Source: CAD feature listing. Evaluate the final solid. Frame: model axes, mm. A direction names the side the tool comes from. Round coordinates to 2 decimals unless told otherwise and drop trailing zeros. Loops run counter-clockwise (first coordinate to the right, second up) from the corner with the lowest first, then second, coordinate; pieces in that order, holes last.
(1) Section D-D, the plane x = 2.5. Return the cut outline in (y, z), plus the area to 3 significant figures.
(2) Section A-A, the plane y = 2. Return the cut outline in (x, z).
(3) Section C-C, the plane y = 3.25. Count the separate pieces of the cut face and the enclosed holes in it, plus the area to 3 significant figures.
(4) Section B-B, the plane z = -0.25. Return the cut outline in (x, y).
(5) Mould query, pull axis Z, two halves, no side actions, for faces 5 (the flat face through (6, 4, 0)), 6 (the flat face through (12, 4, 3)), 7 (the flat face through (1, 0, 3)). Classes: pulls with the +Z half, pulls with the -Z half, needs draft (parallel to the pull), parting line crosses it, or undercut.
(6) First-contact query: pin 1 Ø0.5 at (x, y) = (2.5, 4) entering from +Z; pin 2 Ø3 at (x, y) = (7.5, 6) entering from -Z; pin 3 Ø0.8 at (x, z) = (1, 3.5) entering from -Y. Flat tips, straight axial feed; report the tip coordinate or a pass-through.
(7) Material intervals for probe 1 along Z at (x, y) = (10, 1.25); probe 2 along X at (y, z) = (2, 3.5); probe 3 along Z at (x, y) = (11.5, 6), sorted ascending.
(8) Set-up query: faces 1 (the flat face through (7.2, -0.3, 0.1)), 2 (the flat face through (0, 4, 3)), 3 (the flat face through (12, 0, 3)), 4 (the flat face through (0.5, 4, 3)). Return all of +Z, -Z, +X, -X, +Y, -Y with unobstructed straight access to the full face (end or side cutting, diameter ignored); none if empty.
```python
from build123d import *

# Parameters (mm, degrees)
EXTRUDE_1_DEPTH     = 5.8
SKETCH_2_W          = 11.5
SKETCH_2_H          = 4.8
CUT_EXTRUDE_1_DEPTH = 6
SKETCH_3_W          = 0.6
SKETCH_3_H          = 0.6
EXTRUDE_2_DEPTH     = 6.1
SKETCH_4_W          = 0.6
SKETCH_4_H          = 0.6
EXTRUDE_3_DEPTH     = 7.1
SKETCH_5_W          = 2
SKETCH_5_H          = 4
CUT_EXTRUDE_2_DEPTH = 1


with BuildPart() as part:
    # 草图1 → 凸台-拉伸1 (new body)
    with BuildSketch(Plane.XY):
        Polygon((4, 0), (4, 0.5), (6, 0.5), (6, 0), (6.5, 0), (6.5, 0.5), (8.5, 0.5), (8.5, 0), (9, 0), (9, 0.5), (11, 0.5), (11, 0), (12.5, 0), (12.5, 7), (0, 7), (0, 0), (1.5, 0), (1.5, 0.5), (3.5, 0.5), (3.5, 0), align=None)
    extrude(amount=EXTRUDE_1_DEPTH)

    # 草图2 → 切除-拉伸1 (cut)
    with BuildSketch(Plane(origin=(0, 7, 0), x_dir=(1, 0, 0), z_dir=(0, 1, 0))):
        with Locations((6.25, -2.9)):
            Rectangle(SKETCH_2_W, SKETCH_2_H)
    extrude(amount=-CUT_EXTRUDE_1_DEPTH, mode=Mode.SUBTRACT)

    # 草图3 → 凸台-拉伸2 (add)
    with BuildSketch(Plane.XZ):
        with Locations((5, 3.4)):
            Rectangle(SKETCH_3_W, SKETCH_3_H)
        with Locations((7.5, 3.4)):
            Rectangle(SKETCH_3_W, SKETCH_3_H)
        with Locations((2.5, 3.4)):
            Rectangle(SKETCH_3_W, SKETCH_3_H)
        with Locations((10, 3.4)):
            Rectangle(SKETCH_3_W, SKETCH_3_H)
    extrude(amount=-EXTRUDE_2_DEPTH)

    # 草图4 → 凸台-拉伸3 (add)
    with BuildSketch(Plane.XY.offset(3.7)):
        with Locations((5, -0.3)):
            Rectangle(SKETCH_4_W, SKETCH_4_H)
        with Locations((7.5, -0.3)):
            Rectangle(SKETCH_4_W, SKETCH_4_H)
        with Locations((2.5, -0.3)):
            Rectangle(SKETCH_4_W, SKETCH_4_H)
        with Locations((10, -0.3)):
            Rectangle(SKETCH_4_W, SKETCH_4_H)
    extrude(amount=-EXTRUDE_3_DEPTH)

    # 草图5 → 切除-拉伸2 (cut)
    with BuildSketch(Plane.XY.offset(5.8)):
        with Locations((2.5, 5)):
            Rectangle(SKETCH_5_W, SKETCH_5_H)
        with Locations((10, 5)):
            Rectangle(SKETCH_5_W, SKETCH_5_H)
    extrude(amount=-CUT_EXTRUDE_2_DEPTH, mode=Mode.SUBTRACT)


solid = part.part
```
Output values:
1. outline: (-0.6, -3.4) - (0, -3.4) - (0, 3.1) - (0.5, 3.1) - (0.5, 0) - (7, 0) - (7, 0.5) - (1, 0.5) - (1, 3.1) - (6.1, 3.1) - (6.1, 3.7) - (1, 3.7) - (1, 5.3) - (3, 5.3) - (3, 5.8) - (0.5, 5.8) - (0.5, 3.7) - (-0.6, 3.7) - close
1. area: 14.5 mm2
2. outline: (0, 0) - (12.5, 0) - (12.5, 5.8) - (0, 5.8) - close; (2.2, 3.1) - (2.8, 3.1) - (2.8, 3.7) - (2.2, 3.7) - close; (4.7, 3.1) - (5.3, 3.1) - (5.3, 3.7) - (4.7, 3.7) - close; (7.2, 3.1) - (7.8, 3.1) - (7.8, 3.7) - (7.2, 3.7) - close; (9.7, 3.1) - (10.3, 3.1) - (10.3, 3.7) - (9.7, 3.7) - close; hole (0.5, 0.5) - (12, 0.5) - (12, 5.3) - (0.5, 5.3) - close
3. separate pieces: 6
3. enclosed holes: 0
3. area: 16.7 mm2
4. outline: (2.2, -0.6) - (2.8, -0.6) - (2.8, 0) - (2.2, 0) - close; (4.7, -0.6) - (5.3, -0.6) - (5.3, 0) - (4.7, 0) - close; (7.2, -0.6) - (7.8, -0.6) - (7.8, 0) - (7.2, 0) - close; (9.7, -0.6) - (10.3, -0.6) - (10.3, 0) - (9.7, 0) - close
5. face 5: pulls with the -Z half
5. face 6: undercut
5. face 7: needs draft
6. pin 1: stops at z = 3.7
6. pin 2: stops at z = 0
6. pin 3: stops at y = 0
7. probe 1: z = 0 to 0.5, 3.1 to 3.7, 5.3 to 5.8
7. probe 2: x = 0 to 0.5, 2.2 to 2.8, 4.7 to 5.3, 7.2 to 7.8, 9.7 to 10.3, 12 to 12.5
7. probe 3: z = 0 to 0.5, 5.3 to 5.8
8. face 1: +Z, -Z, -Y
8. face 2: +Z, -Z, -X, +Y, -Y
8. face 3: +Z, -Z, +X, -Y
8. face 4: +Y
